Geometry: see drawing. Coordinates: mm, zero at the bounding-box minimum. A direction names the side the tool comes from. Coordinates: 2 decimals unless noted, no trailing zeros. Write each loop counter-clockwise with the first axis right and the second up, starting at its lowest first coordinate (ties: lowest second). Pieces come first, ordered by that corner, then holes.
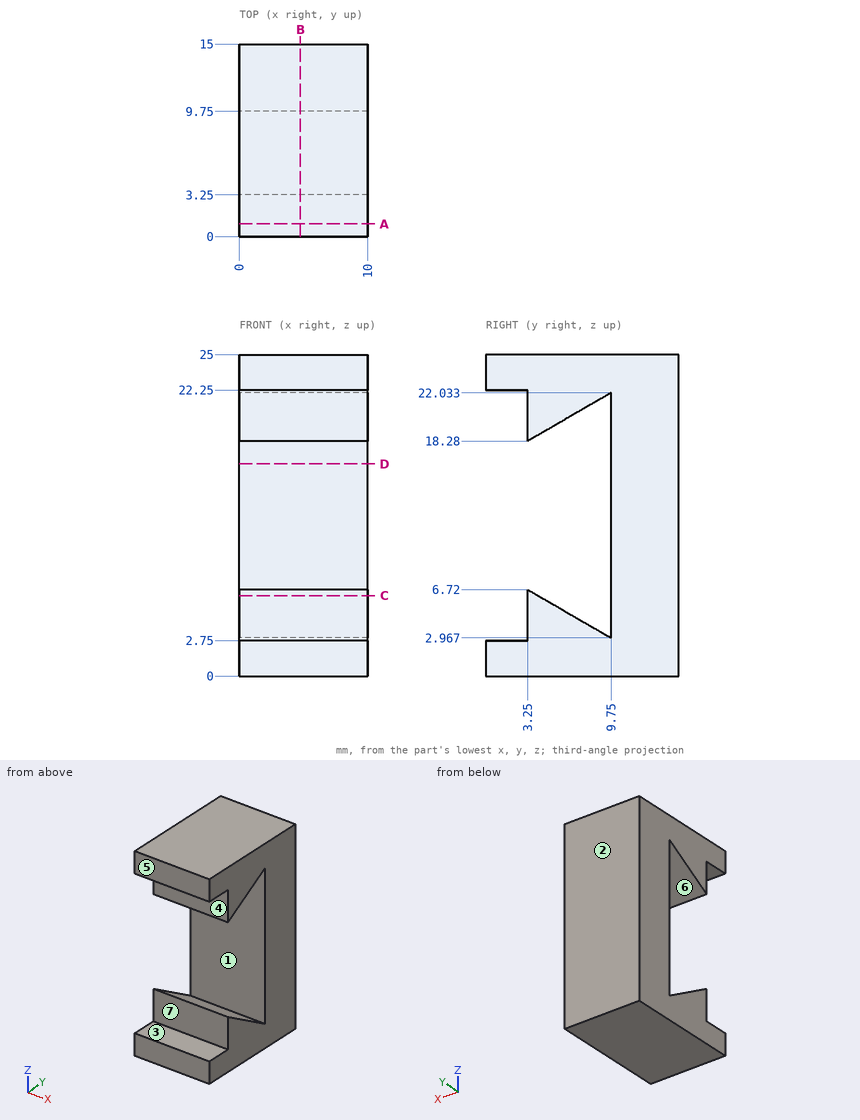
Item 1: Section B-B, the plane x = 4.75. Output: boundary loops of the cut face in (y, z), plus the area to 3 significant figures.
Derived:
outline: (0, 0) - (15, 0) - (15, 25) - (0, 25) - (0, 22.25) - (3.25, 22.25) - (3.25, 18.28) - (9.75, 22.03) - (9.75, 2.97) - (3.25, 6.72) - (3.25, 2.75) - (0, 2.75) - close
area: 212 mm2
Item 2: Pull-direction query (Y, two-part tool) for the marked faces 1, 2, 3 and 4; classes: released by +Y, released by -Y, zero draft, split by the parting line, or undercut.
Derived:
face 1: undercut
face 2: released by +Y
face 3: zero draft
face 4: released by -Y
Item 3: Set-up query: the marked faces 5, 6 and 7. Return all of +Z, -Z, +X, -X, +Y, -Y with unobstructed straight access to the full face (end or side cutting, diameter ignored); none if empty.
Derived:
face 5: +Z, -Z, +X, -X, -Y
face 6: +X, -X
face 7: +X, -X, -Y
Item 4: Material intervals for probe 1 along Z at (x, y) = (7, 2.75); probe 2 along Z at (x, y) = (5.25, 8.5); probe 3 along Y at (x, z) = (5, 6.75), sorted ascending.
Derived:
probe 1: z = 0 to 2.75, 22.25 to 25
probe 2: z = 0 to 3.69, 21.31 to 25
probe 3: y = 9.75 to 15
Item 5: Section A-A, the plane y = 1. Output: boundary loops of the cut face in (x, z).
Derived:
outline: (0, 0) - (10, 0) - (10, 2.75) - (0, 2.75) - close; (0, 22.25) - (10, 22.25) - (10, 25) - (0, 25) - close
Item 6: Pin query (flat end, axial travel): pin 1 (5 mm diameter, centred on x = 7.5, z = 14, fed in from -Y); pin 2 (3 mm diameter, centred on x = 6, z = 4.5, fed in from -Y). Return the tip coordinate at first contact, or that it passes through.
Derived:
pin 1: stops at y = 9.75
pin 2: stops at y = 3.25
Item 7: Section D-D, the plane z = 16.5. Output: boundary loops of the cut face in (x, y).
Derived:
outline: (0, 9.75) - (10, 9.75) - (10, 15) - (0, 15) - close
Item 8: Section C-C, the plane z = 6.25. Output: boundary loops of the cut face in (x, y).
Derived:
outline: (0, 3.25) - (10, 3.25) - (10, 4.06) - (0, 4.06) - close; (0, 9.75) - (10, 9.75) - (10, 15) - (0, 15) - close
